CAD build for the part. Positions are in the model's coordinates, mm. Face numbers are marked on the shaded views. A direction names the side the tool comes from. Round coordinates to 2 decimals unless told otherwise and drop trailing zeros. Loops run counter-clockwise (first coordinate to the right, second up) from the corner with the lowest first, then second, coordinate; pieces in that order, holes last. Notation, with made-up numbers: M -34.5,64 L 0.5,64 A13 cw 0.5,75 Z; hole C 16,69 d3. An arc over 180 degrees is marked long. Put each result on its own line as item: value. Start each with the question number.
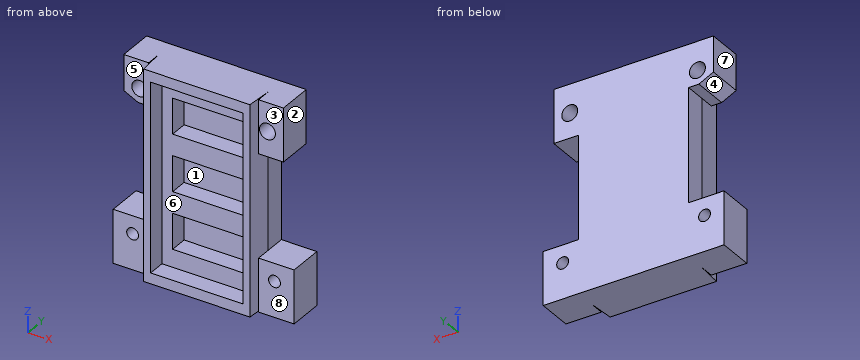
from build123d import *

# Parameters (mm, degrees)
SKETCH1_W           = 26
SKETCH1_H           = 53
SKETCH1_W_2         = 20
SKETCH1_H_2         = 10
BOSS_EXTRUDE1_DEPTH = 5
SKETCH2_W           = 31
SKETCH2_H           = 59
SKETCH2_W_2         = 26
SKETCH2_H_2         = 53
BOSS_EXTRUDE2_DEPTH = 10
SKETCH3_W           = 31
SKETCH3_H           = 59
BOSS_EXTRUDE3_DEPTH = 3
CHAMFER1_SIZE       = 0.5
CHAMFER1_SIZE2      = 7.150333128
SKETCH10_W          = 7
SKETCH10_H          = 15
SKETCH10_R          = 2.25
BOSS_EXTRUDE7_DEPTH = 10
SKETCH11_W          = 7
SKETCH11_H          = 3
CUT_EXTRUDE4_DEPTH  = 10
CHAMFER2_SIZE       = 2
CHAMFER2_SIZE2      = 4.100607683
SKETCH12_W          = 10
SKETCH12_H          = 15
SKETCH12_R          = 1.676379865
BOSS_EXTRUDE8_DEPTH = 10


with BuildPart() as part:
    # Sketch1 → Boss-Extrude1 (new body)
    with BuildSketch(Plane(origin=(0, 0, 0), x_dir=(1, 0, 0), z_dir=(0, 1, 0))):
        with Locations((-13, 26.5)):
            Rectangle(SKETCH1_W, SKETCH1_H)
        with Locations((-13, 27)):
            Rectangle(SKETCH1_W_2, SKETCH1_H_2, mode=Mode.SUBTRACT)
        with Locations((-13, 43)):
            Rectangle(SKETCH1_W_2, SKETCH1_H_2, mode=Mode.SUBTRACT)
        with Locations((-13, 11)):
            Rectangle(SKETCH1_W_2, SKETCH1_H_2, mode=Mode.SUBTRACT)
    extrude(amount=BOSS_EXTRUDE1_DEPTH)

    # Sketch2 → Boss-Extrude2 (add)
    with BuildSketch(Plane(origin=(0, 5, 0), x_dir=(1, 0, 0), z_dir=(0, 1, 0))):
        with Locations((-13, 26.5)):
            Rectangle(SKETCH2_W, SKETCH2_H)
        with Locations((-13, 26.5)):
            Rectangle(SKETCH2_W_2, SKETCH2_H_2, mode=Mode.SUBTRACT)
    extrude(amount=-BOSS_EXTRUDE2_DEPTH)

    # Sketch3 → Boss-Extrude3 (add)
    with BuildSketch(Plane(origin=(0, 5, 0), x_dir=(1, 0, 0), z_dir=(0, 1, 0))):
        with Locations((-13, 26.5)):
            Rectangle(SKETCH3_W, SKETCH3_H)
    extrude(amount=BOSS_EXTRUDE3_DEPTH)

    # Chamfer1
    chamfer1_edges = [part.edges().sort_by_distance(p)[0] for p in [
        (-28.5, -5, -26.5),
        (2.5, -5, -26.5),
    ]]
    chamfer1_side = [part.faces().sort_by_distance(p)[0] for p in [
        (-13, -5, -55.333516692),
    ]]
    chamfer(chamfer1_edges, length=CHAMFER1_SIZE, length2=CHAMFER1_SIZE2, reference=chamfer1_side[0])

    # Sketch10 → Boss-Extrude7 (add)
    with BuildSketch(Plane(origin=(0, 8, 0), x_dir=(1, 0, 0), z_dir=(0, 1, 0))):
        with Locations((6, 4.5)):
            Rectangle(SKETCH10_W, SKETCH10_H)
        with Locations((5, 5)):
            Circle(SKETCH10_R, mode=Mode.SUBTRACT)
        with Locations((-32, 4.5)):
            Rectangle(SKETCH10_W, SKETCH10_H)
        with Locations((-31, 5)):
            Circle(SKETCH10_R, mode=Mode.SUBTRACT)
    extrude(amount=-BOSS_EXTRUDE7_DEPTH)

    # Sketch11 → Cut-Extrude4 (cut)
    with BuildSketch(Plane(origin=(0, 8, 0), x_dir=(1, 0, 0), z_dir=(0, 1, 0))):
        with Locations((-32, 10.5)):
            Rectangle(SKETCH11_W, SKETCH11_H)
    extrude(amount=-CUT_EXTRUDE4_DEPTH, mode=Mode.SUBTRACT)

    # Chamfer2
    chamfer2_edges = [part.edges().sort_by_distance(p)[0] for p in [
        (-35.5, 3, -9),
    ]]
    chamfer2_side = [part.faces().sort_by_distance(p)[0] for p in [
        (-35.5, 3, -3),
    ]]
    chamfer(chamfer2_edges, length=CHAMFER2_SIZE, length2=CHAMFER2_SIZE2, reference=chamfer2_side[0])

    # Sketch12 → Boss-Extrude8 (add)
    with BuildSketch(Plane(origin=(0, 8, 0), x_dir=(1, 0, 0), z_dir=(0, 1, 0))):
        with Locations((7.5, 48.5)):
            Rectangle(SKETCH12_W, SKETCH12_H)
        with Locations((7, 46)):
            Circle(SKETCH12_R, mode=Mode.SUBTRACT)
        with Locations((-33.5, 48.5)):
            Rectangle(SKETCH12_W, SKETCH12_H)
        with Locations((-33, 46)):
            Circle(SKETCH12_R, mode=Mode.SUBTRACT)
    extrude(amount=-BOSS_EXTRUDE8_DEPTH)


solid = part.part
(1) Cut at B-B on z = -5. List the corners of the cut face in (x, y), and give its area (3 significant figures).
(2) Cut at C-C on x = 6. List the corners of the cut face in (y, z), and give its area (3 significant figures).
(3) Cut at A-A on y = 6.5. List the corners of the cut face in (x, z), and give its area (3 significant figures).
(4) Cut at D-D on y = 3.5. Count the separate pieces of the cut face and the enclosed holes in it, and give its area (3 significant figures).
(5) Tool access for the marked faces 4, 5, 6, 7 and 8: list every direction of +Z, -Z, +X, -X, +Y, -Y with a clear straight run to the whole face (end or side of a thin tool).
(6) Drill centre lines: line 1 along Z through (x, y) = (5, 0.75); line 2 along X through (y, z) = (6.25, -46); line 3 along Z through (x, y) = (-4, 2.75). Where is each one in solid material? Low to high.
(7) Mould opens along X. For the marked faces 1, 2 and 3 say: +X half, -X half, draft (parallel to the pull), parting line (faces both ways), or undercut.
(8) Flat gauge pins, fed straight in: pin 1 Ø11 at (x, z) = (8, -51.5) entering from -Y; pin 2 Ø1.5 at (y, z) = (2.5, -27) entering from -X; pin 3 Ø8 at (x, z) = (-17.5, -41.5) entering from -Y. Where does each tip first touch, or does it go through?
Taken from the geometry:
1. outline: M -35.5,-2 L -33.25,-2 L -33.25,8 L -35.5,8 Z; M -28.75,-2 L -28.5,-2 L -28.5,2.15 L -28,-5 L -26,-5 L -26,0 L 0,0 L 0,-5 L 2,-5 L 2.5,2.15 L 2.5,-2 L 2.75,-2 L 2.75,8 L -28.75,8 Z; M 7.25,-2 L 9.5,-2 L 9.5,8 L 7.25,8 Z
1. area: 319 mm2
2. outline: M -2,-56 L 8,-56 L 8,-47.35 L -2,-47.35 Z; M -2,-44.65 L 8,-44.65 L 8,-41 L -2,-41 Z; M -2,-12 L 8,-12 L 8,-7.02 L -2,-7.02 Z; M -2,-2.98 L 8,-2.98 L 8,3 L -2,3 Z
2. area: 233 mm2
3. outline: M -38.5,-56 L 12.5,-56 L 12.5,-41 L 2.5,-41 L 2.5,-12 L 9.5,-12 L 9.5,3 L -35.5,3 L -35.5,-7 L -31.4,-9 L -28.5,-9 L -28.5,-41 L -38.5,-41 Z; hole C -33,-46 d3.35; hole C -31,-5 d4.5; hole C 5,-5 d4.5; hole C 7,-46 d3.35
3. area: 2,260 mm2
4. separate pieces: 1
4. enclosed holes: 7
4. area: 1,660 mm2
5. face 4: -X, +Y, -Y
5. face 5: +Z, -Z, -X, -Y
5. face 6: -Y
5. face 7: +Z, -X, +Y, -Y
5. face 8: +Z, -Z, +X, -Y
6. line 1: -56 to -41, -12 to -7.25, -2.75 to 3
6. line 2: -38.5 to -34.68, -31.32 to 5.32, 8.68 to 12.5
6. line 3: -56 to -48, -38 to -32, -22 to -16, -6 to 3
7. face 1: undercut
7. face 2: +X half
7. face 3: draft
8. pin 1: y = -2
8. pin 2: x = -28.5
8. pin 3: y = 0
